The model under review builds one solid part; all positions refer to its coordinate system, in mm. Face numbers are marked on the shaded views. A direction names the side the tool comes from. Round coordinates to 2 decimals unless told otherwise and drop trailing zeros. Write each loop counter-clockwise with the first axis right and the second up, starting at its lowest first coordinate (ties: lowest second). Pieces come first, ordered by that corner, then holes. Notation, with made-up numbers: (49, -25.5) - (94, -25.5) arc R18 ccw to (94, -18.5) - close; hole circle Ø8 at (-37, -8.5). An arc over 180 degrees is marked (long way). Use one line per item in the form item = value.
from build123d import *

# Parameters (mm, degrees)
F0_R      = 2.159
F0_R_2    = 14.05
F1_DEPTH  = 40
F2_R      = 2.159
F3_DEPTH  = 15
F5_DEPTH  = 25
F6_R      = 2.159
F7_DEPTH  = 25
F4_W      = 19
F4_H      = 20
F4_R      = 2.159
F8_DEPTH  = 25
F9_R      = 2.159
F10_DEPTH = 57.1
F11_R     = 3.5
F12_DEPTH = 20
F9_W      = 4.5
F9_H      = 20
F13_DEPTH = 25
F14_DEPTH = 50


# Not quite as in the source:
# - an extrude ends at something that could not be found from the text; its depth is read off the source's solid


with BuildPart() as f1:
    # F0 (on Front) → F1 (new body)
    with BuildSketch(Plane.XZ):
        Polygon((30, -5.94), (30, 22.5), (-30, 22.5), (-30, -5.94), (-13.44, -22.5), (13.44, -22.5), align=None)
        with Locations((-13.44, -15.94)):
            Circle(F0_R, mode=Mode.SUBTRACT)
        with Locations((-19, -2.5)):
            Circle(F0_R, mode=Mode.SUBTRACT)
        with Locations((13.44, -15.94)):
            Circle(F0_R, mode=Mode.SUBTRACT)
        with Locations((0, -2.5)):
            Circle(F0_R_2, mode=Mode.SUBTRACT)
        with Locations((19, -2.5)):
            Circle(F0_R, mode=Mode.SUBTRACT)
        with Locations((-13.44, 10.94)):
            Circle(F0_R, mode=Mode.SUBTRACT)
        with Locations((13.44, 10.94)):
            Circle(F0_R, mode=Mode.SUBTRACT)
    extrude(amount=F1_DEPTH)

    # F2 (on face) → F3 (cut)
    with BuildSketch(Plane.XY.offset(22.5)):
        with Locations((-22.5, -7)):
            Circle(F2_R)
        with Locations((22.5, -7)):
            Circle(F2_R)
        with Locations((-22.5, -33)):
            Circle(F2_R)
        with Locations((22.5, -33)):
            Circle(F2_R)
    extrude(amount=-F3_DEPTH, mode=Mode.SUBTRACT)

    # F2 (on face) → F5 (join)
    with BuildSketch(Plane.XY.offset(22.5)):
        with Locations((22.5, -33)):
            Circle(F2_R)
    extrude(amount=-F5_DEPTH)

    # F6 (on face) → F7 (join)
    with BuildSketch(Plane.XY.offset(22.5)):
        with Locations((22.5, -7)):
            Circle(F6_R)
        with Locations((22.5, -33)):
            Circle(F6_R)
        with Locations((-22.5, -7)):
            Circle(F6_R)
        with Locations((-22.5, -33)):
            Circle(F6_R)
    extrude(amount=-F7_DEPTH)

    # F4 (on face) → F8 (join)
    with BuildSketch(Plane.XY.offset(22.5)):
        with Locations((20.5, -30)):
            Rectangle(F4_W, F4_H)
        with Locations((22.5, -33)):
            Circle(F4_R, mode=Mode.SUBTRACT)
    extrude(amount=F8_DEPTH)

    # F9 (on face) → F10 (join)
    with BuildSketch(Plane.XY.offset(47.5)):
        with Locations((22.5, -33)):
            Circle(F9_R)
    extrude(amount=-F10_DEPTH)

    # F11 (on face) → F12 (join, through all)
    with BuildSketch(Plane.XZ.offset(40)):
        Polygon((11, 83.5), (11, 47.5), (30, 47.5), (30, -5.94), (91, 55.06), (91, 97.5), (11, 97.5), align=None)
        with Locations((29, 61)):
            Circle(F11_R, mode=Mode.SUBTRACT)
        with Locations((29, 83.5)):
            Circle(F11_R, mode=Mode.SUBTRACT)
        with Locations((74, 61)):
            Circle(F11_R, mode=Mode.SUBTRACT)
        with Locations((74, 83.5)):
            Circle(F11_R, mode=Mode.SUBTRACT)
    extrude(amount=-F12_DEPTH)

    # F9 (on face) → F13 (join)
    with BuildSketch(Plane.XY.offset(47.5)):
        with Locations((8.75, -30)):
            Rectangle(F9_W, F9_H)
    extrude(amount=-F13_DEPTH)

    # F9 (on face) → F14 (join, through all)
    with BuildSketch(Plane.XY.offset(47.5)):
        with Locations((8.75, -30)):
            Rectangle(F9_W, F9_H)
    extrude(amount=F14_DEPTH)


solid = f1.part
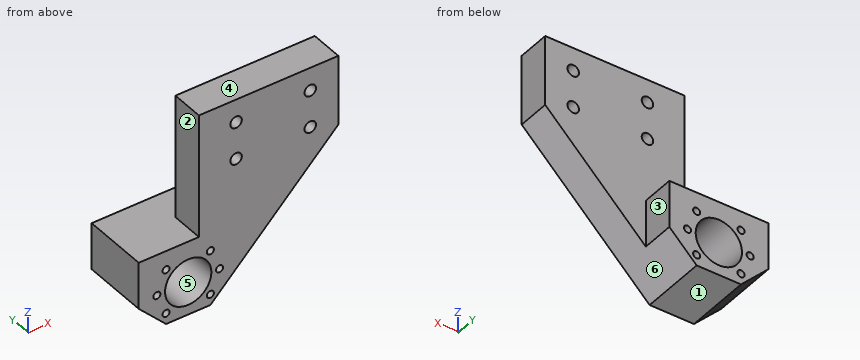
(1) Insertion check: P1, Ø10, axis at x = 52, y = -31, coming from the -Z side; P2, Ø5, axis at x = 23.5, y = -11, coming from the -Z side; P3, Ø2.5, axis at x = -13.44, z = -15.94, coming from the +Y side; P4, Ø9, axis at x = 74, z = 61, coming from the +Y side. Each pin has a flat end and moves straight along its axis. Give the tip position at first contact, or say it passes through.
Geometry results:
P1 = 11.06
P2 = -14.94
P3 = through
P4 = -20
(2) The part is to be moulded in two halves that separate along X. For the marked faces 4, 5 and 6, say which applies: +X half, -X half, draft (parallel to the pull), parting line (faces both ways), or undercut.
Geometry results:
face_4 = draft
face_5 = undercut
face_6 = +X half
(3) Machinability: for the marked faces 1, 2 and 3, which of the approach directions +Z, -Z, +X, -X, +Y, -Y give a long, thin tool a straight path to every point of the face, cutting with its end or side? Answer none if there is none.
Geometry results:
face_1 = -Z, +X, -X, +Y, -Y
face_2 = +Z, -X, +Y, -Y
face_3 = +Z, -Z, +X, +Y
(4) Add section D-D on x = 28. Write out the cut boundary in (y, z), then the cut area to 3 significant figures.
Geometry results:
outline = (-40, -7.94) - (0, -7.94) - (0, 22.5) - (-20, 22.5) - (-20, 57.65) - (-40, 57.65) - close; (-40, 64.35) - (-20, 64.35) - (-20, 80.15) - (-40, 80.15) - close; (-40, 86.85) - (-20, 86.85) - (-20, 97.5) - (-40, 97.5) - close
area = 2,450 mm2
(5) To check wall thickness, follow L1, parallel to Z at x = 29, y = -25.75; L2, parallel to X at y = -19, z = 10; L3, parallel to X at y = -37, z = 62. State the ranges of each line that lie inside material, in increasing order.
Geometry results:
L1 = -6.94 to 57.5, 64.5 to 80, 87 to 97.5
L2 = -30 to -15.38, -11.5 to -6.42, 6.42 to 11.5, 15.38 to 30
L3 = 6.5 to 25.65, 32.35 to 70.65, 77.35 to 91
(6) Add section A-A on x = 0. Write out the cut boundary in (y, z).
Geometry results:
outline = (-40, -22.5) - (0, -22.5) - (0, -16.55) - (-40, -16.55) - close; (-40, 11.55) - (0, 11.55) - (0, 22.5) - (-40, 22.5) - close
(7) Add section B-B on z = 61. Write out the cut boundary in (x, y), then the cut area to 3 significant figures.
Geometry results:
outline = (6.5, -40) - (25.5, -40) - (25.5, -20) - (6.5, -20) - close; (32.5, -40) - (70.5, -40) - (70.5, -20) - (32.5, -20) - close; (77.5, -40) - (91, -40) - (91, -20) - (77.5, -20) - close
area = 1,410 mm2
(8) Add section C-C on y = -7. Write out the cut boundary in (x, z), then the cut area to 3 significant figures.
Geometry results:
outline = (-30, -5.94) - (-13.44, -22.5) - (13.44, -22.5) - (30, -5.94) - (30, 22.5) - (-30, 22.5) - close; hole (-21.16, -2.5) arc R2.16 ccw (long way) to (-20.34, -0.81) - (-20.34, -2.5) - close; hole circle Ø4.32 at (-13.44, -15.94); hole circle Ø4.32 at (-13.44, 10.94); hole circle Ø28.1 at (0, -2.5); hole circle Ø4.32 at (13.44, -15.94); hole circle Ø4.32 at (13.44, 10.94); hole (20.34, -2.5) - (20.34, -0.81) arc R2.16 ccw (long way) to (21.16, -2.5) - close
area = 1,720 mm2
